Can you work these out from the model? Positions are in its coordinate system, mm. A direction names the side the tool comes from. Coordinates: 2 decimals unless noted, no trailing zeros. Order: outer loops, then holes, each group sorted by start corner. A loop starts at its lowest first (then second) coordinate and runs counter-clockwise, first axis right, second up. Notation, with made-up numbers: (79.5, 43.5) - (137.5, 43.5) arc R36 cw to (137.5, 79.5) - close; hole circle Ø1 at (84, 30.25). An arc over 180 degrees is marked (long way). Use a Markdown table: item, result. Add a question column.
(1) For pin 1 Ø5 at (y, z) = (25.5, -3) entering from +X; pin 2 Ø12 at (x, y) = (-15, 21) entering from -Z; pin 3 Ø3 at (x, z) = (-14.5, -6) entering from +Y, each with a flat end and sliding along its axis, tell me the tip position at first contact or that it passes through.
(2) I want a section at A-A (y = -1). List the corners of the cut face in (x, z) for me, and give its area (3 significant figures).
(3) If I drill on L1, parallel to Z at x = -2.5, y = 34; L2, parallel to Y at x = 2, z = -3.75; L3, parallel to Y at x = -17.5, z = 2.5, over which ranges is the centre line in solid material (lowest first)? Write a range as [from, to].
(4) On a 3-axis mill with a long thin cutter (end or side, diameter ignored), from which of +Z, -Z, +X, -X, +Y, -Y can I reach the whole of each face in a straight line? I mean faces 1 (the flat face through (0, 20, 0)), 2 (the flat face through (-30, 14, 1)). Say none if no direction works.
(5) I want a section at D-D (y = 13.5). List the corners of the cut face in (x, z) for me.
(6) I want a section at B-B (x = 10). List the corners of the cut face in (y, z) for me, and give its area (3 significant figures).
(7) I want a section at C-C (z = 1). List the corners of the cut face in (x, y) for me.
```python
from build123d import *

# Parameters (mm, degrees)
F0_W     = 60
F0_H     = 40
F1_DEPTH = 5
F2_SIZE  = 8
F3_W     = 60
F3_H     = 9
F3_H_2   = 5
F4_DEPTH = 4
F5_SIZE  = 3
F6_SIZE2 = 8.6602540378
F6_SIZE  = 5
F7_R     = 1
F8_W     = 85.4819267988
F8_H     = 62.53941264
F9_DEPTH = 1


with BuildPart() as f1:
    # F0 (on Top) → F1 (new body)
    with BuildSketch(Plane.XY):
        with Locations((0, 20)):
            Rectangle(F0_W, F0_H)
    extrude(amount=F1_DEPTH)

    # F2
    f2_edges = [f1.edges().sort_by_distance(p)[0] for p in [
        (30, 40, 2.5),
        (-30, 40, 2.5),
    ]]
    chamfer(f2_edges, length=F2_SIZE)

    # F3 (on face) → F4 (join)
    with BuildSketch(Plane.XZ):
        with Locations((0, -4.5)):
            Rectangle(F3_W, F3_H)
        with Locations((0, 2.5)):
            Rectangle(F3_W, F3_H_2)
    extrude(amount=F4_DEPTH)

    # F5
    f5_edges = [f1.edges().sort_by_distance(p)[0] for p in [
        (-30, 14, 5),
        (30, 14, 5),
        (0, 40, 5),
        (26, 36, 5),
        (-26, 36, 5),
    ]]
    chamfer(f5_edges, length=F5_SIZE)

    # F6
    f6_edges = [f1.edges().sort_by_distance(p)[0] for p in [
        (-30, -2, -9),
        (30, -2, -9),
    ]]
    f6_side = f1.faces().sort_by_distance((0, -2, -9))[0]
    chamfer(f6_edges, length=F6_SIZE, length2=F6_SIZE2, reference=f6_side)

    # F7
    f7_edges = [f1.edges().sort_by_distance(p)[0] for p in [
        (0, -4, -9),
    ]]
    fillet(f7_edges, radius=F7_R)

    # F8 (on face) → F9 (cut)
    with BuildSketch(Plane.XY.offset(5)):
        with Locations((-1.7423257232, 24.269700516)):
            Rectangle(F8_W, F8_H)
        Polygon((27, -4), (-27, -4), (-27, 30.7573593129), (-20.7573593129, 37), (20.7573593129, 37), (27, 30.7573593129), align=None, mode=Mode.SUBTRACT)
        Polygon((-27, 30.7573593129), (-27, -4), (27, -4), (27, 30.7573593129), (20.7573593129, 37), (-20.7573593129, 37), align=None)
    extrude(amount=-F9_DEPTH, mode=Mode.SUBTRACT)


solid = f1.part
```
Answers follow:
| question | item | result |
|---|---|---|
| 1 | pin 1 | passes through |
| 1 | pin 2 | stops at z = 0 |
| 1 | pin 3 | stops at y = 0 |
| 2 | outline | (-30, -0.34) - (-25, -9) - (25, -9) - (30, -0.34) - (30, 2) - (28, 4) - (-28, 4) - (-30, 2) - close |
| 2 | area | 733 mm² |
| 3 | L1 | z = [0, 4] |
| 3 | L2 | y = [-4, 0] |
| 3 | L3 | y = [-4, 39.5] |
| 4 | face 1 | -Z, +X, -X, +Y |
| 4 | face 2 | +Z, -Z, -X, +Y, -Y |
| 5 | outline | (-30, 0) - (30, 0) - (30, 2) - (28, 4) - (-28, 4) - (-30, 2) - close |
| 6 | outline | (-4, -8) arc R1 ccw to (-3, -9) - (0, -9) - (0, 0) - (40, 0) - (40, 2) - (38, 4) - (-4, 4) - close |
| 6 | area | 210 mm² |
| 7 | outline | (-30, -4) - (30, -4) - (30, 32) - (22, 40) - (-22, 40) - (-30, 32) - close |
